```python
from build123d import *

# Parameters (mm, degrees)
MAIN_SKETCH_W                         = 73.5
MAIN_SKETCH_H                         = 45.5
MAIN_SKETCH_W_2                       = 8.85
MAIN_SKETCH_H_2                       = 31.2
MAIN_SKETCH_R                         = 2.2479
LIP_DEPTH                             = 3.175
MOUNTING_BASE_OUTLINE_W               = 63.5
MOUNTING_BASE_OUTLINE_H               = 35.5
MOUNTING_BASE_OUTLINE_R               = 2.2479
MOUNTING_BASE_OUTLINE_R_2             = 4
MOUNTING_BASE_DEPTH                   = 11
HEATER_CART_4_40_TAPS_D               = 2.2606
HEATER_CART_4_40_TAPS_DEPTH           = 7.595
HEATER_CART_4_40_TAPS_TIP             = 0.679152758
HEATER_CART_4_40_TAPS_ON_FACE_2_D     = 2.2606
HEATER_CART_4_40_TAPS_ON_FACE_2_DEPTH = 7.595
HEATER_CART_4_40_TAPS_ON_FACE_2_TIP   = 0.679152758
MAIN_SKETCH_12_W                      = 8.85
MAIN_SKETCH_12_H                      = 31.2
MAIN_SKETCH_12_R                      = 0.285
BOTTOM_SQUARE_CUTOUT_DEPTH            = 2
SQUARE_MICRO_D_CUTOUT_START           = 5.3
SQUARE_MICRO_D_CUTOUT_OUTLINE_W       = 8.85
SQUARE_MICRO_D_CUTOUT_OUTLINE_H       = 31.2
SQUARE_MICRO_D_CUTOUT_OUTLINE_R       = 0.285
SQUARE_MICRO_D_CUTOUT_DEPTH           = 5.7
SKETCH15_W                            = 8.067488146
SKETCH15_H                            = 23.070933647
CUT_EXTRUDE1_DEPTH                    = 11
INTERNAL_CORNER_CUTOUTS_FILLET_R      = 2
CHIP_CLAMP_0_80_TAPS_AT_2_COUNT       = 2
CHIP_CLAMP_0_80_TAPS_AT_2_PITCH       = 17.1232
CHIP_CLAMP_0_80_TAPS_AT_3_COUNT       = 2
CHIP_CLAMP_0_80_TAPS_AT_3_PITCH       = 17.1232
F_2_56_CLOSE_CLEAR_43_0_089_D         = 2.2606
PCB_2_56_TAPS_D                       = 1.778
PCB_2_56_TAPS_DEPTH                   = 5.734
PCB_2_56_TAPS_TIP                     = 0.53416509
BOTTOM_COVER_2_56_TAPS_D              = 1.778
BOTTOM_COVER_2_56_TAPS_DEPTH          = 5.734
BOTTOM_COVER_2_56_TAPS_TIP            = 0.53416509
F_2_56_TAPPED_HOLE1_D                 = 1.778
F_2_56_TAPPED_HOLE1_DEPTH             = 5.734
F_2_56_TAPPED_HOLE1_TIP               = 0.53416509


# Read off the part's stored shape, not the designer's step: Mounting_Base, Square_Micro_D_Cutout
with BuildPart() as part:
    # Main_Sketch → Lip (new body)
    with BuildSketch(Plane(origin=(0, 0, 0), x_dir=(1, 0, 0), z_dir=(0, 1, 0))):
        with Locations((36.75, -22.75)):
            Rectangle(MAIN_SKETCH_W, MAIN_SKETCH_H)
        with Locations((10.925, -22.749999985)):
            Rectangle(MAIN_SKETCH_W_2, MAIN_SKETCH_H_2, mode=Mode.SUBTRACT)
        with Locations(Location((18.75, -22.75, 0), (0, 0, 270))):
            Circle(MAIN_SKETCH_R, mode=Mode.SUBTRACT)
        with BuildLine():
            ThreePointArc((31.675, -20.175), (29.907233047, -15.907233047), (34.175, -17.675))
            Line((34.175, -17.675), (39.325, -17.675))
            ThreePointArc((39.325, -17.675), (43.592766953, -15.907233047), (41.825, -20.175))
            Line((41.825, -20.175), (41.825, -25.325))
            ThreePointArc((41.825, -25.325), (43.592766953, -29.592766953), (39.325, -27.825))
            Line((39.325, -27.825), (34.175, -27.825))
            ThreePointArc((34.175, -27.825), (29.907233047, -29.592766953), (31.675, -25.325))
            Line((31.675, -25.325), (31.675, -20.175))
        make_face(mode=Mode.SUBTRACT)
        with Locations(Location((54.75, -22.75, 0), (0, 0, 270))):
            Circle(MAIN_SKETCH_R, mode=Mode.SUBTRACT)
    extrude(amount=LIP_DEPTH)

    # Mounting_Base outline → Mounting_Base (add)
    with BuildSketch(Plane(origin=(0, 0, 0), x_dir=(1, 0, 0), z_dir=(0, 1, 0))):
        with Locations((36.75, -22.75)):
            Rectangle(MOUNTING_BASE_OUTLINE_W, MOUNTING_BASE_OUTLINE_H)
        with Locations((18.75, -22.75)):
            Circle(MOUNTING_BASE_OUTLINE_R, mode=Mode.SUBTRACT)
        with Locations((54.75, -22.75)):
            Circle(MOUNTING_BASE_OUTLINE_R, mode=Mode.SUBTRACT)
        with Locations((36.75, -22.75)):
            Circle(MOUNTING_BASE_OUTLINE_R_2, mode=Mode.SUBTRACT)
    extrude(amount=MOUNTING_BASE_DEPTH)

    # Heater_Cart_#4-40_Taps
    with Locations(Plane(origin=(52.725, 7.825, 5), x_dir=(-1, 0, 0), z_dir=(0, 0, -1))):
        with Locations((0, 0), (31.95, 0)):
            Hole(HEATER_CART_4_40_TAPS_D / 2, depth=HEATER_CART_4_40_TAPS_DEPTH)
            with Locations((0, 0, -(HEATER_CART_4_40_TAPS_DEPTH + HEATER_CART_4_40_TAPS_TIP / 2))):  # 118° drill point
                Cone(0, HEATER_CART_4_40_TAPS_D / 2, HEATER_CART_4_40_TAPS_TIP, mode=Mode.SUBTRACT)

    # Heater_Cart_#4-40_Taps on face 2
    with Locations(Plane(origin=(20.775, 7.825, 40.5), x_dir=(1, 0, 0), z_dir=(0, 0, 1))):
        with Locations((0, 0), (31.95, 0)):
            Hole(HEATER_CART_4_40_TAPS_ON_FACE_2_D / 2, depth=HEATER_CART_4_40_TAPS_ON_FACE_2_DEPTH)
            with Locations((0, 0, -(HEATER_CART_4_40_TAPS_ON_FACE_2_DEPTH + HEATER_CART_4_40_TAPS_ON_FACE_2_TIP / 2))):  # 118° drill point
                Cone(0, HEATER_CART_4_40_TAPS_ON_FACE_2_D / 2, HEATER_CART_4_40_TAPS_ON_FACE_2_TIP, mode=Mode.SUBTRACT)

    # Main_Sketch<12> → Bottom_square_cutout (cut)
    # profile 1 of 2: a face of its own
    with BuildSketch(Plane(origin=(0, 0, 0), x_dir=(1, 0, 0), z_dir=(0, 1, 0))):
        with Locations((10.925, -22.749999985)):
            Rectangle(MAIN_SKETCH_12_W, MAIN_SKETCH_12_H)
        with BuildLine():
            ThreePointArc((10.385689992, -35.285466808), (9.155254643, -35.471894814), (7.986136174, -35.045410869))
            ThreePointArc((7.986136174, -35.045410869), (7.18175843, -34.143309058), (6.891255927, -32.970099985))
            Line((6.891255927, -32.970099985), (6.891255927, -12.529899985))
            ThreePointArc((6.891255927, -12.529899985), (7.18175845, -11.356690961), (7.986136174, -10.454589189))
            ThreePointArc((7.986136174, -10.454589189), (9.155254643, -10.028105244), (10.385689992, -10.21453325))
            Line((10.385689992, -10.21453325), (13.424612074, -11.500982853))
            ThreePointArc((13.424612074, -11.500982853), (14.540409069, -12.427601581), (14.958744073, -13.816349588))
            Line((14.958744073, -13.816349588), (14.958744073, -31.683650456))
            ThreePointArc((14.958744073, -31.683650456), (14.540409073, -33.072398471), (13.424612074, -33.999017205))
            Line((13.424612074, -33.999017205), (10.385689992, -35.285466808))
        make_face(mode=Mode.SUBTRACT)
    # profile 2 of 2: a face of its own
    with BuildSketch(Plane(origin=(0, 0, 0), x_dir=(1, 0, 0), z_dir=(0, 1, 0))):
        with BuildLine():
            ThreePointArc((7.986136174, -35.045410869), (7.18175843, -34.143309058), (6.891255927, -32.970099985))
            Line((6.891255927, -32.970099985), (6.891255927, -12.529899985))
            ThreePointArc((6.891255927, -12.529899985), (7.18175845, -11.356690961), (7.986136174, -10.454589189))
            ThreePointArc((7.986136174, -10.454589189), (9.155254643, -10.028105244), (10.385689992, -10.21453325))
            Line((10.385689992, -10.21453325), (13.424612074, -11.500982853))
            ThreePointArc((13.424612074, -11.500982853), (14.540409069, -12.427601581), (14.958744073, -13.816349588))
            Line((14.958744073, -13.816349588), (14.958744073, -31.683650456))
            ThreePointArc((14.958744073, -31.683650456), (14.540409073, -33.072398471), (13.424612074, -33.999017205))
            Line((13.424612074, -33.999017205), (10.385689992, -35.285466808))
            ThreePointArc((10.385689992, -35.285466808), (9.155254643, -35.471894814), (7.986136174, -35.045410869))
        make_face()
        with Locations(Location((10.239255927, -22.75, 0), (0, 0, 270))):
            Circle(MAIN_SKETCH_12_R, mode=Mode.SUBTRACT)
    bottom_square_cutout = extrude(amount=BOTTOM_SQUARE_CUTOUT_DEPTH, mode=Mode.SUBTRACT)

    # Square_Micro_D_Cutout outline → Square_Micro_D_Cutout (cut)
    with BuildSketch(Plane(origin=(0, 0, 0), x_dir=(1, 0, 0), z_dir=(0, 1, 0)).offset(SQUARE_MICRO_D_CUTOUT_START)):
        with Locations((10.925, -22.749999985)):
            Rectangle(SQUARE_MICRO_D_CUTOUT_OUTLINE_W, SQUARE_MICRO_D_CUTOUT_OUTLINE_H)
        with Locations((10.239255927, -22.75)):
            Circle(SQUARE_MICRO_D_CUTOUT_OUTLINE_R, mode=Mode.SUBTRACT)
    square_micro_d_cutout = extrude(amount=SQUARE_MICRO_D_CUTOUT_DEPTH, mode=Mode.SUBTRACT)

    # Sketch15 → Cut-Extrude1 (cut)
    with BuildSketch(Plane(origin=(0, 0, 0), x_dir=(1, 0, 0), z_dir=(0, 1, 0))):
        with Locations((10.925, -22.749999985)):
            Rectangle(SKETCH15_W, SKETCH15_H)
    cut_extrude1 = extrude(amount=CUT_EXTRUDE1_DEPTH, mode=Mode.SUBTRACT)

    # MicroD_Mirror: Bottom_square_cutout, Square_Micro_D_Cutout, Cut-Extrude1 across plane
    add(bottom_square_cutout.mirror(Plane(origin=(36.75, 0, 0), x_dir=(0, 0, 1), z_dir=(1, 0, 0))), mode=Mode.SUBTRACT)
    add(square_micro_d_cutout.mirror(Plane(origin=(36.75, 0, 0), x_dir=(0, 0, 1), z_dir=(1, 0, 0))), mode=Mode.SUBTRACT)
    add(cut_extrude1.mirror(Plane(origin=(36.75, 0, 0), x_dir=(0, 0, 1), z_dir=(1, 0, 0))), mode=Mode.SUBTRACT)

    # Internal_Corner_cutouts_fillet
    internal_corner_cutouts_fillet_edges = [part.edges().sort_by_distance(p)[0] for p in [
        (15.35, 1, 38.349999985),
        (15.35, 1, 7.149999985),
        (6.5, 1, 7.149999985),
        (6.5, 1, 38.349999985),
        (15.35, 8.15, 38.349999985),
        (6.5, 8.15, 38.349999985),
        (6.5, 8.15, 7.149999985),
        (15.35, 8.15, 7.149999985),
        (14.958744073, 3.65, 34.285466808),
        (14.958744073, 3.65, 11.214533161),
        (6.891255927, 3.65, 11.214533161),
        (6.891255927, 3.65, 34.285466808),
        (58.15, 1, 7.149999985),
        (58.15, 1, 38.349999985),
        (67, 1, 38.349999985),
        (67, 1, 7.149999985),
        (67, 8.15, 7.149999985),
        (67, 8.15, 38.349999985),
        (58.15, 8.15, 38.349999985),
        (58.15, 8.15, 7.149999985),
        (58.541255927, 3.65, 11.214533161),
        (58.541255927, 3.65, 34.285466808),
        (66.608744073, 3.65, 34.285466808),
        (66.608744073, 3.65, 11.214533161),
    ]]
    fillet(internal_corner_cutouts_fillet_edges, radius=INTERNAL_CORNER_CUTOUTS_FILLET_R)

    # Sketch3 → Chip_Clamp_#0-80 Taps (revolve, cut)
    with BuildSketch(Plane(origin=(36.75, 11, 31.3116), x_dir=(0, 0, 1), z_dir=(1, 0, 0))):
        Polygon((0, 0), (0, 4.358890611), (0.59563, 4.001), (0.59563, 0), align=None)
    chip_clamp_0_80_taps = revolve(axis=Axis((36.75, 17.35, 31.3116), (0, -1, 0)), mode=Mode.SUBTRACT)

    # Chip_Clamp_#0-80 Taps at 2: Chip_Clamp_#0-80 Taps ×2
    with Locations(*[(0, 0, -i * CHIP_CLAMP_0_80_TAPS_AT_2_PITCH) for i in range(1, CHIP_CLAMP_0_80_TAPS_AT_2_COUNT)]):
        add(chip_clamp_0_80_taps, mode=Mode.SUBTRACT)

    # Chip_Clamp_#0-80 Taps at 3: Chip_Clamp_#0-80 Taps ×2
    with Locations(*[(0, 0, -i * CHIP_CLAMP_0_80_TAPS_AT_3_PITCH) for i in range(1, CHIP_CLAMP_0_80_TAPS_AT_3_COUNT)]):
        add(chip_clamp_0_80_taps, mode=Mode.SUBTRACT)

    # 2-56_Close_Clear#43 (0.089) (through all)
    with Locations(Plane(origin=(18.375, 0, 43), x_dir=(0, 0, -1), z_dir=(0, -1, 0))):
        with Locations((0, 0), (40.5, 0), (40.5, 36.75), (0, 36.75)):
            Hole(F_2_56_CLOSE_CLEAR_43_0_089_D / 2)

    # PCB #2-56 Taps
    with Locations(Plane(origin=(17.75, 11, 14.25), x_dir=(0, 0, 1), z_dir=(0, 1, 0))):
        with Locations((0, 0), (17, 0), (0, 38), (17, 38)):
            Hole(PCB_2_56_TAPS_D / 2, depth=PCB_2_56_TAPS_DEPTH)
            with Locations((0, 0, -(PCB_2_56_TAPS_DEPTH + PCB_2_56_TAPS_TIP / 2))):  # 118° drill point
                Cone(0, PCB_2_56_TAPS_D / 2, PCB_2_56_TAPS_TIP, mode=Mode.SUBTRACT)

    # Bottom_Cover#2-56 Taps
    with Locations(Plane(origin=(54.75, 0, 18.75), x_dir=(0, 0, -1), z_dir=(0, -1, 0))):
        with Locations((0, 0), (-8, 0), (-8, -36), (0, -36)):
            Hole(BOTTOM_COVER_2_56_TAPS_D / 2, depth=BOTTOM_COVER_2_56_TAPS_DEPTH)
            with Locations((0, 0, -(BOTTOM_COVER_2_56_TAPS_DEPTH + BOTTOM_COVER_2_56_TAPS_TIP / 2))):  # 118° drill point
                Cone(0, BOTTOM_COVER_2_56_TAPS_D / 2, BOTTOM_COVER_2_56_TAPS_TIP, mode=Mode.SUBTRACT)

    # #2-56 Tapped Hole1
    with Locations(Plane(origin=(32.94, 0, 31.38), x_dir=(0, 0, -1), z_dir=(0, -1, 0))):
        with Locations((0, 0), (-7.62, 0), (-7.62, 7.62), (0, 7.62)):
            Hole(F_2_56_TAPPED_HOLE1_D / 2, depth=F_2_56_TAPPED_HOLE1_DEPTH)
            with Locations((0, 0, -(F_2_56_TAPPED_HOLE1_DEPTH + F_2_56_TAPPED_HOLE1_TIP / 2))):  # 118° drill point
                Cone(0, F_2_56_TAPPED_HOLE1_D / 2, F_2_56_TAPPED_HOLE1_TIP, mode=Mode.SUBTRACT)


solid = part.part
```
The model under review builds one solid part; all positions refer to its coordinate system, in mm. A direction names the side the tool comes from. Give positions to 0.01 mm unless a question says otherwise; leave off trailing zeros. Answer in a Markdown table with one row per item. Add a question column.
1. Wall thickness on line 1 along X through (y, z) = (6, 22.75); line 2 along X through (y, z) = (1.25, 36); line 3 along X through (y, z) = (1.3, 2.5): over which ranges is each line inside the solid? List them lowest first. Write a range as [from, to].
2. Draft analysis for pull direction X (two halves, no side actions). For faces 1 (the flat face through (36, 0, 17)), 2 (the cylindrical face through (19.5, 2.91, 27.23)), state which applies: +X half, -X half, draft (parallel to the pull), parting line (faces both ways), or undercut.
3. We need section A-A on y = 10. State how many separate pieces and enclosed holes the cut face has, then the cut area to 3 significant figures.
4. Insertion check: P1, Ø3.5, axis at y = 3, z = 21, coming from the -X side; P2, Ø4, axis at x = 31, y = 10, coming from the -Z side; P3, Ø6, axis at y = 7.5, z = 7.5, coming from the -X side; P4, Ø1.8, axis at x = 20.775, y = 7.825, coming from the -Z side. Each pin has a flat end and moves straight along its axis. Give the tip position at first contact, or say it passes through.
5. Tool access review of faces 3 (the flat face through (6.5, 1, 23)), 4 (the flat face through (63, 8, 7.15)), 5 (the flat face through (58.541, 4, 23)): name each direction out of +Z, -Z, +X, -X, +Y, -Y from which nothing blocks a thin tool from reaching the whole face with its end or side.
Ans:
| question | item | result |
|---|---|---|
| 1 | line 1 | x = [5, 6.5], [15.35, 16.5], [21, 32.75], [40.75, 52.5], [57, 58.15], [67, 68.5] |
| 1 | line 2 | x = [0, 6.5], [15.35, 58.15], [67, 73.5] |
| 1 | line 3 | x = [0, 17.24], [19.51, 53.99], [56.26, 73.5] |
| 2 | face 1 | draft |
| 2 | face 2 | undercut |
| 3 | separate pieces | 1 |
| 3 | enclosed holes | 11 |
| 3 | area | 1,610 mm^2 |
| 4 | P1 | stops at x = 0 |
| 4 | P2 | stops at z = 5 |
| 4 | P3 | stops at x = 5 |
| 4 | P4 | stops at z = 12.73 |
| 5 | face 3 | -Y |
| 5 | face 4 | +Y |
| 5 | face 5 | +Y, -Y |
